```python
from build123d import *

# Parameters (mm, degrees)
SKETCH1_W           = 45
SKETCH1_H           = 35
BOSS_EXTRUDE1_DEPTH = 300
FILLET1_R           = 8
SHELL1_T            = -3
SKETCH3_R           = 7.45
SKETCH3_R_2         = 6.45
BOSS_EXTRUDE2_DEPTH = 103
SKETCH4_R           = 10.65
SKETCH4_R_2         = 6.45
BOSS_EXTRUDE3_DEPTH = 25


with BuildPart() as part:
    # Sketch1 → Boss-Extrude1 (new body)
    with BuildSketch(Plane(origin=(0, 0, 0), x_dir=(0, 0, -1), z_dir=(1, 0, 0))):
        Rectangle(SKETCH1_W, SKETCH1_H)
    extrude(amount=BOSS_EXTRUDE1_DEPTH)

    # Fillet1
    fillet1_edges = [part.edges().sort_by_distance(p)[0] for p in [
        (150, -17.5, -22.5),
        (150, -17.5, 22.5),
    ]]
    fillet(fillet1_edges, radius=FILLET1_R)

    # Shell1
    shell1_openings = [part.faces().sort_by_distance(p)[0] for p in [
        (150, 17.5, 0),
    ]]
    offset(amount=SHELL1_T, openings=shell1_openings, kind=Kind.INTERSECTION)

    # Sketch3 → Boss-Extrude2 (add)
    with BuildSketch(Plane(origin=(290, 0, 0), x_dir=(0, 0, -1), z_dir=(1, 0, 0))):
        Circle(SKETCH3_R)
        Circle(SKETCH3_R_2, mode=Mode.SUBTRACT)
    extrude(amount=BOSS_EXTRUDE2_DEPTH)

    # Sketch4 → Boss-Extrude3 (add)
    with BuildSketch(Plane(origin=(393, 0, 0), x_dir=(0, 0, -1), z_dir=(1, 0, 0))):
        Circle(SKETCH4_R)
        Circle(SKETCH4_R_2, mode=Mode.SUBTRACT)
    extrude(amount=BOSS_EXTRUDE3_DEPTH)


solid = part.part
```
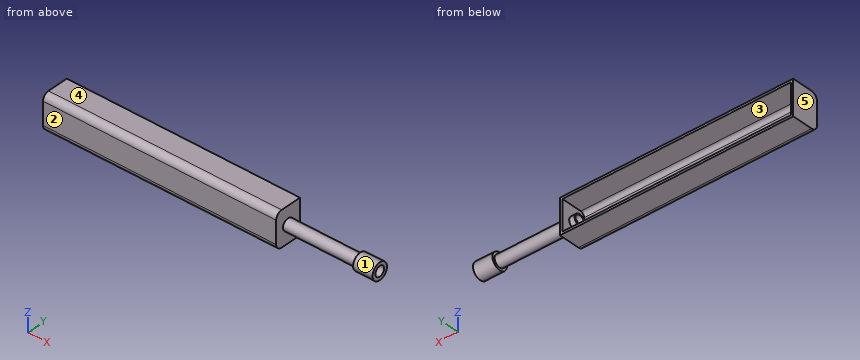
CAD build for the part. Positions are in the model's coordinates, mm. Face numbers are marked on the shaded views. A direction names the side the tool comes from. Coordinates: 2 decimals unless noted, no trailing zeros. Order: outer loops, then holes, each group sorted by start corner. A loop starts at its lowest first (then second) coordinate and runs counter-clockwise, first axis right, second up. Notation, with made-up numbers: M 23,-5 L 65,-5 A13 cw 65,14 Z; hole C 60,13.25 d5. An arc over 180 degrees is marked long. Answer as CSV lines item,"result".
1) Drill centre lines: L1, parallel to Y at x = 295, z = 0; L2, parallel to Z at x = 295.25, y = 0; L3, parallel to X at y = 11, z = 3.5. Where is each one in solid material? Low to high. Write a range as from..to.
Verdict:
L1,"-17.5..-14.5, -7.45..-6.45, 6.45..7.45"
L2,"-22.5..-19.5, -7.45..-6.45, 6.45..7.45, 19.5..22.5"
L3,"0..3, 297..300"
2) Flat gauge pins, fed straight in: P1, Ø23, axis at x = 87, z = -2, coming from the +Y side; P2, Ø10.5, axis at y = 0, z = 0, coming from the +X side; P3, Ø5, axis at y = -9.5, z = 0, coming from the -X side; P4, Ø5, axis at x = 144, y = -13.5, coming from the -Z side. Where does each tip first touch, or does it go through?
Verdict:
P1,"y = -14.5"
P2,"x = 300"
P3,"x = 0"
P4,"z = -22.36"
3) Cut at A-A (y = 0). List the corners of the cut face in (x, z), then the cut area to 3 significant figures.
Verdict:
outline,"M 0,-22.5 L 300,-22.5 L 300,-7.45 L 393,-7.45 L 393,-10.65 L 418,-10.65 L 418,-6.45 L 300,-6.45 L 300,6.45 L 418,6.45 L 418,10.65 L 393,10.65 L 393,7.45 L 300,7.45 L 300,22.5 L 0,22.5 Z; hole M 3,-19.5 L 297,-19.5 L 297,-7.45 L 290,-7.45 L 290,-6.45 L 297,-6.45 L 297,6.45 L 290,6.45 L 290,7.45 L 297,7.45 L 297,19.5 L 3,19.5 Z"
area,"2,440 mm2"
4) Cut at B-B (z = 0). List the corners of the cut face in (x, y).
Verdict:
outline,"M 0,-17.5 L 300,-17.5 L 300,-7.45 L 393,-7.45 L 393,-10.65 L 418,-10.65 L 418,-6.45 L 300,-6.45 L 300,6.45 L 418,6.45 L 418,10.65 L 393,10.65 L 393,7.45 L 300,7.45 L 300,17.5 L 297,17.5 L 297,7.45 L 290,7.45 L 290,6.45 L 297,6.45 L 297,-6.45 L 290,-6.45 L 290,-7.45 L 297,-7.45 L 297,-14.5 L 3,-14.5 L 3,17.5 L 0,17.5 Z"
5) Cut at C-C (x = 102.5). List the corners of the cut face in (y, z), then the cut area to 3 significant figures.
Verdict:
outline,"M -17.5,-14.5 A8 ccw -9.5,-22.5 L 17.5,-22.5 L 17.5,-19.5 L -9.5,-19.5 A5 cw -14.5,-14.5 L -14.5,14.5 A5 cw -9.5,19.5 L 17.5,19.5 L 17.5,22.5 L -9.5,22.5 A8 ccw -17.5,14.5 Z"
area,"310 mm2"
6) 3-axis set-ups, long thin cutter, end or side, ignore diameter. For the marked faces 1 and 2: which of +Z, -Z, +X, -X, +Y, -Y reach the whole face in a straight line?
Verdict:
face 1,"+X"
face 2,"+Z, -Z, +X, -X, -Y"
7) Cut at D-D (x = 312). List the corners of the cut face in (y, z).
Verdict:
outline,"C 0,0 d14.9; hole C 0,0 d12.9"
8) Mould opens along X. For the marked faces 3, 4 and 5 say: released by +X, released by -X, zero draft, split by the parting line, or undercut.
Verdict:
face 3,"undercut"
face 4,"zero draft"
face 5,"released by -X"
